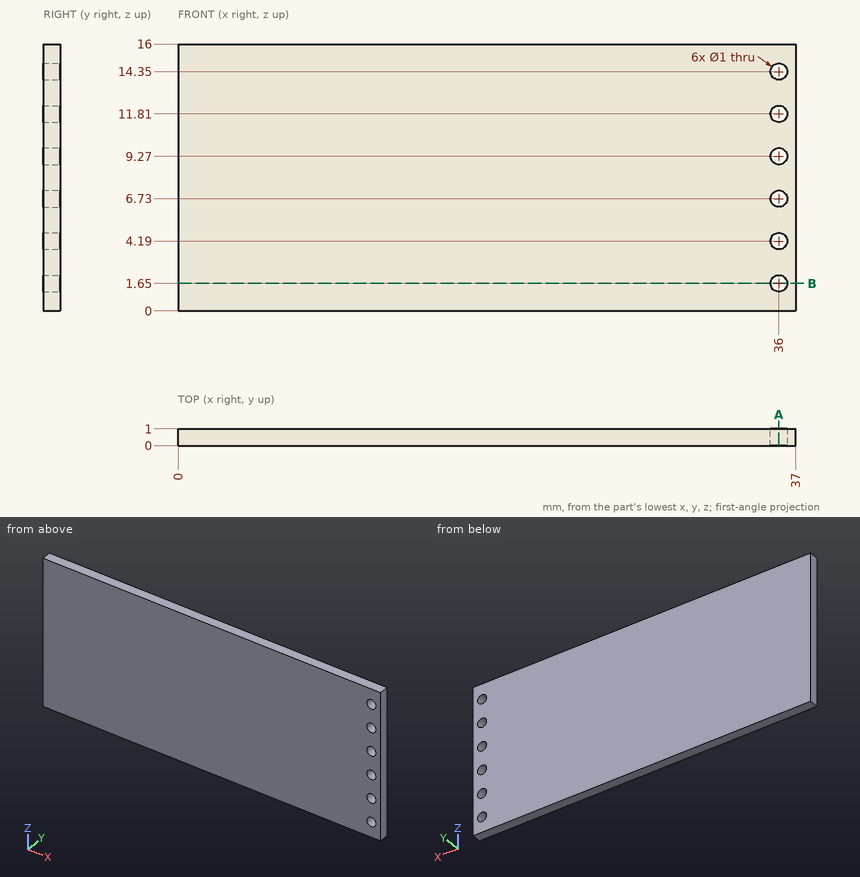
Check sheet for the drawn part. Datum: minimum x, y, z corner. Units: mm. Give positions to 0.01 mm unless a question says otherwise; leave off trailing zeros. Order: outer loops, then holes, each group sorted by start corner. A loop starts at its lowest first (then second) coordinate and runs counter-clockwise, first axis right, second up. Notation, with made-up numbers: (42.25, -3) - (76.25, -3) arc R17 ccw to (76.25, 23) - close; hole circle Ø5 at (14, 36). An arc over 180 degrees is marked (long way). Write item = value, one per line. Start each with the question number.
1) Section check A-A (x = 36). Enter the section's corners in (y, z), then the cut area to 3 significant figures.
2) Section check B-B (z = 1.65). Enter the section's corners in (x, y), then the cut area to 3 significant figures.
3) Scan lines: L1, parallel to X at y = 0.55, z = 11.75; L2, parallel to X at y = 0.1, z = 9.5. Record each from-to range of solid material in increasing order.
Geometry check:
q1.outline = (0, 0) - (1, 0) - (1, 1.15) - (0, 1.15) - close; (0, 2.15) - (1, 2.15) - (1, 3.69) - (0, 3.69) - close; (0, 4.69) - (1, 4.69) - (1, 6.23) - (0, 6.23) - close; (0, 7.23) - (1, 7.23) - (1, 8.77) - (0, 8.77) - close; (0, 9.77) - (1, 9.77) - (1, 11.31) - (0, 11.31) - close; (0, 12.31) - (1, 12.31) - (1, 13.85) - (0, 13.85) - close; (0, 14.85) - (1, 14.85) - (1, 16) - (0, 16) - close
q1.area = 10.0 mm2
q2.outline = (0, 0) - (35.5, 0) - (35.5, 1) - (0, 1) - close; (36.5, 0) - (37, 0) - (37, 1) - (36.5, 1) - close
q2.area = 36.0 mm2
q3.L1 = 0 to 35.5, 36.5 to 37
q3.L2 = 0 to 35.56, 36.44 to 37
